from build123d import *

# Parameters (mm, degrees)
SKETCH_1_W           = 35
SKETCH_1_H           = 20
EXTRUDE_1_DEPTH      = 8
SKETCH_2_W           = 29
SKETCH_2_H           = 14
CUT_EXTRUDE_2_DEPTH  = 0.8
SKETCH_3_W           = 29
SKETCH_3_H           = 7.2
CUT_EXTRUDE_4_DEPTH  = 42.097445176
SKETCH_4_W           = 6
SKETCH_4_H           = 6
CUT_EXTRUDE_5_DEPTH  = 42.097445176
SKETCH_5_R           = 1.2
CUT_EXTRUDE_6_DEPTH  = 42.097445176
CUT_EXTRUDE_START    = 8
CUT_EXTRUDE_8_DEPTH  = 2.3
SKETCH_6_R           = 2.2
CUT_EXTRUDE_10_DEPTH = 2


with BuildPart() as part:
    # 草圖1 → 填料-伸長1 (new body)
    with BuildSketch(Plane(origin=(0, 0, 0), x_dir=(1, 0, 0), z_dir=(0, 1, 0))):
        with Locations((17.5, 10)):
            Rectangle(SKETCH_1_W, SKETCH_1_H)
    extrude(amount=EXTRUDE_1_DEPTH)

    # 草圖2 → 除料-伸長2 (cut)
    with BuildSketch(Plane(origin=(0, 0, 0), x_dir=(1, 0, 0), z_dir=(0, 1, 0))):
        with Locations((20.5, 7)):
            Rectangle(SKETCH_2_W, SKETCH_2_H)
    extrude(amount=CUT_EXTRUDE_2_DEPTH, mode=Mode.SUBTRACT)

    # 草圖3 → 除料-伸長4 (cut, through all)
    with BuildSketch(Plane(origin=(0, 0, 0), x_dir=(1, 0, 0), z_dir=(0, 1, 0))):
        with Locations((20.5, 3.6)):
            Rectangle(SKETCH_3_W, SKETCH_3_H)
    extrude(amount=CUT_EXTRUDE_4_DEPTH, mode=Mode.SUBTRACT)

    # 草圖4 → 除料-伸長5 (cut, through all)
    with BuildSketch(Plane(origin=(0, 0, 0), x_dir=(1, 0, 0), z_dir=(0, 1, 0))):
        with Locations((32, 17)):
            Rectangle(SKETCH_4_W, SKETCH_4_H)
    extrude(amount=CUT_EXTRUDE_5_DEPTH, mode=Mode.SUBTRACT)

    # 草圖5 → 除料-伸長6 (cut, through all)
    with BuildSketch(Plane(origin=(0, 0, 0), x_dir=(1, 0, 0), z_dir=(0, 1, 0))):
        with Locations(Location((3, 16, 0), (0, 0, 270))):
            Circle(SKETCH_5_R)
        with Locations(Location((3, 4, 0), (0, 0, 270))):
            Circle(SKETCH_5_R)
        with Locations(Location((9, 16, 0), (0, 0, 270))):
            Circle(SKETCH_5_R)
        with Locations(Location((26, 16, 0), (0, 0, 270))):
            Circle(SKETCH_5_R)
    extrude(amount=CUT_EXTRUDE_6_DEPTH, mode=Mode.SUBTRACT)

    # 草圖7 → 除料-伸長8 (cut)
    with BuildSketch(Plane(origin=(0, 0, 0), x_dir=(1, 0, 0), z_dir=(0, 1, 0)).offset(CUT_EXTRUDE_START)):
        Polygon((26, 18.4), (23.921539031, 17.2), (23.921539031, 14.8), (26, 13.6), (28.078460969, 14.8), (28.078460969, 17.2), align=None)
        Polygon((9, 18.4), (6.921539031, 17.2), (6.921539031, 14.8), (9, 13.6), (11.078460969, 14.8), (11.078460969, 17.2), align=None)
    extrude(amount=-CUT_EXTRUDE_8_DEPTH, mode=Mode.SUBTRACT)

    # 草圖6 → 除料-伸長10 (cut)
    with BuildSketch(Plane(origin=(0, 0, 0), x_dir=(1, 0, 0), z_dir=(0, 1, 0))):
        with Locations(Location((3, 16, 0), (0, 0, 90))):
            Circle(SKETCH_6_R)
        with Locations(Location((3, 4, 0), (0, 0, 90))):
            Circle(SKETCH_6_R)
    extrude(amount=CUT_EXTRUDE_10_DEPTH, mode=Mode.SUBTRACT)


solid = part.part
Can you work these out from the model? Positions are in its coordinate system, mm. A direction names the side the tool comes from. Give positions to 0.01 mm unless a question says otherwise; leave off trailing zeros. Loops run counter-clockwise (first coordinate to the right, second up) from the corner with the lowest first, then second, coordinate; pieces in that order, holes last. Notation, with made-up numbers: (72.25, 24) - (101.25, 24) arc R26 ccw to (101.25, 60) - close; hole circle Ø4 at (46, -10.75). An arc over 180 degrees is marked (long way). One line per item, written item: value.
(1) I need wall thicknesses on line 1 along X through (y, z) = (0.75, -16); line 2 along Z through (x, y) = (3, 4.8); line 3 along X through (y, z) = (3.55, -16). Which ranges of each line are inside material? Lowest first, please.
Verdict:
line 1: 0 to 0.8, 5.2 to 7.8, 10.2 to 24.8, 27.2 to 29
line 2: -20 to -17.2, -14.8 to -5.2, -2.8 to 0
line 3: 0 to 1.8, 4.2 to 7.8, 10.2 to 24.8, 27.2 to 29
(2) I'm going to push flat-ended pins straight in: pin 1 (3 mm diameter, centred on x = 3, z = -4, fed in from -Y); pin 2 (3.5 mm diameter, centred on x = 19, z = -12, fed in from -Y); pin 3 (2.5 mm diameter, centred on y = 7, z = -16, fed in from +X). Where does each tip first touch, or does it pass through?
Verdict:
pin 1: y = 2
pin 2: y = 0.8
pin 3: x = 29
(3) If we section it at B-B, the plane y = 3: List the corners of the cut face in (x, z) for me.
Verdict:
outline: (0, -20) - (29, -20) - (29, -14) - (35, -14) - (35, -7.2) - (6, -7.2) - (6, 0) - (0, 0) - close; hole circle Ø2.4 at (3, -16); hole circle Ø2.4 at (3, -4); hole circle Ø2.4 at (9, -16); hole circle Ø2.4 at (26, -16)
(4) If we mould it in two halves opening along X, with no side actions, what happens to faces 1 (the face through (29, 4, -17)), 2 (the face through (11.078, 7, -16)), 3 (the face through (20, 4, -7.2))? For each: released by +X, released by -X, zero draft, split by the parting line, or undercut.
Verdict:
face 1: released by +X
face 2: undercut
face 3: zero draft
(5) On a 3-axis mill with a long thin cutter (end or side, diameter ignored), from which of +Z, -Z, +X, -X, +Y, -Y can I reach the whole of each face in a straight line? I mean faces 4 (the face through (28.078, 7, -16)), 5 (the face through (2.34, 0.99, -18.1)), 6 (the face through (14, 4, -20)), 7 (the face through (20, 0.8, -11)). Say none if no direction works.
Verdict:
face 4: +Y
face 5: -Y
face 6: -Z, +X, -X, +Y, -Y
face 7: +Z, +X, -Y
(6) If we section it at C-C, the plane x = 3: List the corners of the cut face in (y, z) for me, plus the area to 3 significant figures.
Verdict:
outline: (0, -20) - (8, -20) - (8, -17.2) - (2, -17.2) - (2, -18.2) - (0, -18.2) - close; (0, -13.8) - (2, -13.8) - (2, -14.8) - (8, -14.8) - (8, -5.2) - (2, -5.2) - (2, -6.2) - (0, -6.2) - close; (0, -1.8) - (2, -1.8) - (2, -2.8) - (8, -2.8) - (8, 0) - (0, 0) - close
area: 114 mm^2
(7) If we section it at A-A, the plane z = -4: List the corners of the cut face in (x, y) for me.
Verdict:
outline: (0, 0) - (0.8, 0) - (0.8, 2) - (1.8, 2) - (1.8, 8) - (0, 8) - close; (4.2, 2) - (5.2, 2) - (5.2, 0) - (6, 0) - (6, 8) - (4.2, 8) - close
(8) If we section it at D-D, the plane z = -16: List the corners of the cut face in (x, y) for me.
Verdict:
outline: (0, 0) - (0.8, 0) - (0.8, 2) - (1.8, 2) - (1.8, 8) - (0, 8) - close; (4.2, 2) - (5.2, 2) - (5.2, 0) - (7.8, 0) - (7.8, 5.7) - (6.92, 5.7) - (6.92, 8) - (4.2, 8) - close; (10.2, 0) - (24.8, 0) - (24.8, 5.7) - (23.92, 5.7) - (23.92, 8) - (11.08, 8) - (11.08, 5.7) - (10.2, 5.7) - close; (27.2, 0) - (29, 0) - (29, 8) - (28.08, 8) - (28.08, 5.7) - (27.2, 5.7) - close
